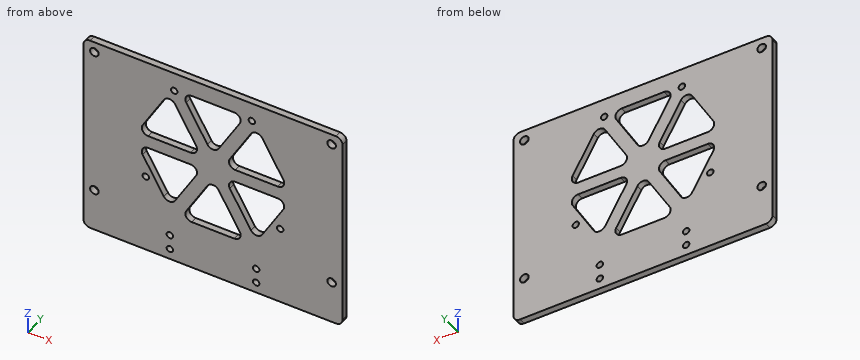
from build123d import *

# Parameters (mm, degrees)
SKETCH_1_W          = 120
SKETCH_1_H          = 80
EXTRUDE_1_DEPTH     = 3
SKETCH_3_R          = 1.5
CUT_EXTRUDE_2_DEPTH = 4
SKETCH_4_R          = 2
CUT_EXTRUDE_3_DEPTH = 4
SKETCH_5_W          = 120
SKETCH_5_H          = 3
EXTRUDE_2_DEPTH     = 15
CUT_EXTRUDE_4_DEPTH = 15
FILLET_1_R          = 3
SKETCH_7_R          = 1.5
CUT_EXTRUDE_5_DEPTH = 4
FILLET_2_R          = 3


with BuildPart() as part:
    # 草图1 → 凸台-拉伸1 (new body)
    with BuildSketch(Plane(origin=(0, 0, 0), x_dir=(1, 0, 0), z_dir=(0, 1, 0))):
        Rectangle(SKETCH_1_W, SKETCH_1_H)
    extrude(amount=EXTRUDE_1_DEPTH)

    # 草图3 → 切除-拉伸2 (cut, through all)
    with BuildSketch(Plane(origin=(0, 3, 0), x_dir=(1, 0, 0), z_dir=(0, 1, 0))):
        with Locations((-31.176914536, 18)):
            Circle(SKETCH_3_R)
        with Locations((31.176914536, 18)):
            Circle(SKETCH_3_R)
        with Locations((-18, -31.176914536)):
            Circle(SKETCH_3_R)
        with Locations((18, -31.176914536)):
            Circle(SKETCH_3_R)
    extrude(amount=-CUT_EXTRUDE_2_DEPTH, mode=Mode.SUBTRACT)

    # 草图4 → 切除-拉伸3 (cut, through all)
    with BuildSketch(Plane(origin=(0, 3, 0), x_dir=(1, 0, 0), z_dir=(0, 1, 0))):
        with Locations((-55, 35)):
            Circle(SKETCH_4_R)
        with Locations((55, 35)):
            Circle(SKETCH_4_R)
        with Locations((55, -35)):
            Circle(SKETCH_4_R)
        with Locations((-55, -35)):
            Circle(SKETCH_4_R)
    extrude(amount=-CUT_EXTRUDE_3_DEPTH, mode=Mode.SUBTRACT)

    # 草图5 → 凸台-拉伸2 (add)
    with BuildSketch(Plane(origin=(0, 0, -40), x_dir=(-1, 0, 0), z_dir=(0, 0, -1))):
        with Locations((0, 1.5)):
            Rectangle(SKETCH_5_W, SKETCH_5_H)
    extrude(amount=EXTRUDE_2_DEPTH)

    # 草图6 → 切除-拉伸4 (cut)
    with BuildSketch(Plane(origin=(0, 3, 0), x_dir=(1, 0, 0), z_dir=(0, 1, 0))):
        Polygon((-15.011106999, 32), (0, 6), (15.011106999, 32), align=None)
        Polygon((5.196152423, 3), (35.218366421, 3), (20.207259422, 29), align=None)
        Polygon((5.196152423, -3), (20.207259422, -29), (35.218366421, -3), align=None)
        Polygon((-15.011106999, -32), (15.011106999, -32), (0, -6), align=None)
        Polygon((-35.218366421, -3), (-20.207259422, -29), (-5.196152423, -3), align=None)
        Polygon((-35.218366421, 3), (-5.196152423, 3), (-20.207259422, 29), align=None)
    extrude(amount=-CUT_EXTRUDE_4_DEPTH, mode=Mode.SUBTRACT)

    # 圆角1
    fillet_1_edges = [part.edges().sort_by_distance(p)[0] for p in [
        (35.218366421, 1.5, -3),
        (5.196152423, 1.5, -3),
        (20.207259422, 1.5, -29),
        (-20.207259422, 1.5, -29),
        (-5.196152423, 1.5, -3),
        (-35.218366421, 1.5, -3),
        (15.011106999, 1.5, -32),
        (0, 1.5, -6),
        (-15.011106999, 1.5, -32),
        (-15.011106999, 1.5, 32),
        (0, 1.5, 6),
        (15.011106999, 1.5, 32),
        (-35.218366421, 1.5, 3),
        (-5.196152423, 1.5, 3),
        (-20.207259422, 1.5, 29),
        (20.207259422, 1.5, 29),
        (5.196152423, 1.5, 3),
        (35.218366421, 1.5, 3),
    ]]
    fillet(fillet_1_edges, radius=FILLET_1_R)

    # 草图7 → 切除-拉伸5 (cut, through all)
    with BuildSketch(Plane(origin=(0, 3, 0), x_dir=(1, 0, 0), z_dir=(0, 1, 0))):
        with Locations((-20, 50)):
            Circle(SKETCH_7_R)
        with Locations((20, 50)):
            Circle(SKETCH_7_R)
        with Locations((-20, 43)):
            Circle(SKETCH_7_R)
        with Locations((20, 43)):
            Circle(SKETCH_7_R)
    extrude(amount=-CUT_EXTRUDE_5_DEPTH, mode=Mode.SUBTRACT)

    # 圆角2
    fillet_2_edges = [part.edges().sort_by_distance(p)[0] for p in [
        (60, 1.5, -55),
        (-60, 1.5, -55),
        (60, 1.5, 40),
        (-60, 1.5, 40),
    ]]
    fillet(fillet_2_edges, radius=FILLET_2_R)


solid = part.part
Input: part model. Units: mm. Frame: model coordinates. Round coordinates to 2 decimals unless told otherwise and drop trailing zeros. Loops run counter-clockwise (first coordinate to the right, second up) from the corner with the lowest first, then second, coordinate; pieces in that order, holes last. Notation, with made-up numbers: (46, 15.25) -> (64, 15.25) arc R34 ccw to (64, 51.25) -> close; hole circle Ø9 at (58, 77.25). An arc over 180 degrees is marked (long way). Answer as a JSON object with one key per item and string values. Group by question number.
1) Section query A-A on z = -50. Output: boundary loops of the cut face in (x, y), plus the area to 3 significant figures.
2) Section query D-D on y = 0.6. State how many separate pieces and enclosed holes the cut face has, plus the area to 3 significant figures.
3) Section query B-B on x = 55. Output: boundary loops of the cut face in (y, z), plus the area to 3 significant figures.
4) Pin query (flat end, axial travel): pin 1 (3.5 mm diameter, centred on x = 18, z = 31.18, fed in from -Y). Return the tip coordinate at first contact, or that it passes through.
5) Ray query, L1, parallel to Z at x = 20, y = 1.6; L2, parallel to X at y = 0.8, z = 35; L3, parallel to Z at x = 55, y = 1.6. Return the intervals inside material, ascending.
6) Section query C-C on z = -18. Output: boundary loops of the cut face in (x, y).
Reply:
{
 "1": {"outline": "(-60, 0) -> (-21.5, 0) -> (-21.5, 3) -> (-60, 3) -> close; (-18.5, 0) -> (18.5, 0) -> (18.5, 3) -> (-18.5, 3) -> close; (21.5, 0) -> (60, 0) -> (60, 3) -> (21.5, 3) -> close", "area": "342 mm2"},
 "2": {"separate pieces": "1", "enclosed holes": "18", "area": "9,050 mm2"},
 "3": {"outline": "(0, -55) -> (3, -55) -> (3, -37) -> (0, -37) -> close; (0, -33) -> (3, -33) -> (3, 33) -> (0, 33) -> close; (0, 37) -> (3, 37) -> (3, 40) -> (0, 40) -> close", "area": "261 mm2"},
 "4": {"pin 1": "stops at y = 0"},
 "5": {"L1": "z = -55 to -51.5, -48.5 to -44.5, -41.5 to -25.99, -3 to 3, 25.99 to 40", "L2": "x = -60 to -57, -53 to 53, 57 to 60", "L3": "z = -55 to -37, -33 to 33, 37 to 40"},
 "6": {"outline": "(-60, 0) -> (-32.68, 0) -> (-32.68, 3) -> (-60, 3) -> close; (-29.68, 0) -> (-26.56, 0) -> (-26.56, 3) -> (-29.68, 3) -> close; (-13.86, 0) -> (-6.93, 0) -> (-6.93, 3) -> (-13.86, 3) -> close; (6.93, 0) -> (13.86, 0) -> (13.86, 3) -> (6.93, 3) -> close; (26.56, 0) -> (29.68, 0) -> (29.68, 3) -> (26.56, 3) -> close; (32.68, 0) -> (60, 0) -> (60, 3) -> (32.68, 3) -> close"}
}
